Input: part model. Units: mm. Frame: model coordinates. Face numbers are marked on the shaded views. A direction names the side the tool comes from. Give positions to 0.01 mm unless a question says otherwise; leave off trailing zeros. Write each loop counter-clockwise with the first axis right and the second up, starting at its lowest first coordinate (ties: lowest second). Pieces come first, ordered by that corner, then holes. Notation, with made-up numbers: (43, 60.5) - (56, 60.5) arc R24 cw to (56, 70.5) - close; hole circle Ø7 at (-36, 83.5). An arc over 180 degrees is marked (long way). Use a Markdown table: item, result. Add a question column.
1. Set-up query: the marked faces 1 and 2. Return all of +Z, -Z, +X, -X, +Y, -Y with unobstructed straight access to the full face (end or side cutting, diameter ignored); none if empty.
2. Pin query (flat end, axial travel): pin 1 (10.5 mm diameter, centred on x = -90.93, y = 52.5, fed in from +Z); pin 2 (5 mm diameter, centred on x = 50.5, z = 10.5, fed in from -Y); pin 3 (17 mm diameter, centred on x = 0, y = 105, fed in from +Z); pin 4 (4 mm diameter, centred on y = -31.5, z = 7.5, fed in from +X). Return the tip coordinate at first contact, or that it passes through.
3. Section query B-B, the plane x = -91. Return loops of the section in (y, z).
4. Section query D-D, the plane z = 1. Return loops of the section in (x, y), plus the area to 3 significant figures.
5. Mould query, pull axis X, two halves, no side actions, for the marked faces 3, 4 and 5. Classes: released by +X, released by -X, zero draft, split by the parting line, or undercut.
6. Section query C-C, the plane y = -105. Return loops of the section in (x, z), plus the area to 3 significant figures.
7. Material intervals for probe 1 along Y at (x, z) = (0, -1.75); probe 2 along Z at (x, y) = (-73.5, 66.5); probe 3 along Z at (x, y) = (-5, 78.5), sorted ascending.
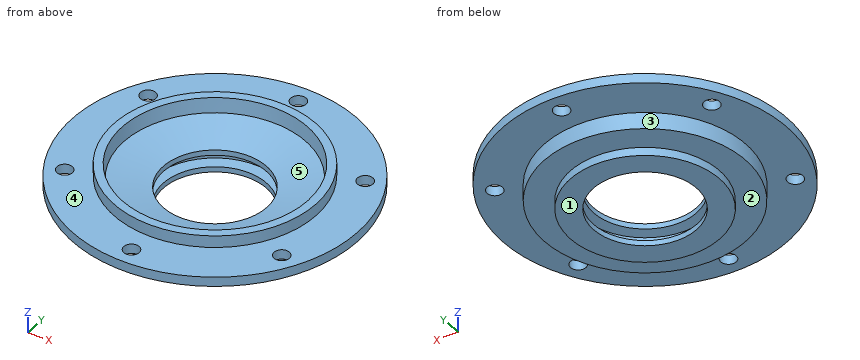
```python
from build123d import *

# Parameters (mm, degrees)
SKETCH_2_R               = 6.5
CUT_EXTRUDE_1_DEPTH      = 172
PATTERN_CIRCULAR_1_COUNT = 6


with BuildPart() as part:
    # 草图1 → 旋转1 (revolve)
    with BuildSketch(Plane(origin=(0, 0, 0), x_dir=(0, 0, -1), z_dir=(1, 0, 0)), mode=Mode.PRIVATE) as revolve_1_sk:
        Polygon((-9.5, 43.5), (-5, 43.5), (-4, 52.5), (4, 52.5), (5, 43.5), (9.5, 43.5), (9.5, 63), (2.5, 63), (2.5, 85), (-11.5, 85), (-11.5, 120), (-19.5, 120), (-19.5, 85), (-29.5, 85), (-29.5, 78), (-17.5, 76.5), align=None)
    revolve(revolve_1_sk.sketch.rotate(Axis((0, 0, 1000), (0, 0, -1)), 90), axis=Axis((0, 0, 1000), (0, 0, -1)))

    # 草图2 → 切除-拉伸1 (cut, through all)
    with BuildSketch(Plane(origin=(0, 0, 11.5), x_dir=(-1, 0, 0), z_dir=(0, 0, -1))):
        with Locations((0, 105)):
            Circle(SKETCH_2_R)
    cut_extrude_1 = extrude(amount=-CUT_EXTRUDE_1_DEPTH, mode=Mode.SUBTRACT)

    # 阵列(圆周)1: 切除-拉伸1 ×6 about axis
    pattern_circular_1_axis = Axis((0, 0, 0), (0, 0, 1))
    for i in range(1, PATTERN_CIRCULAR_1_COUNT):
        add(cut_extrude_1.rotate(pattern_circular_1_axis, i * 360 / PATTERN_CIRCULAR_1_COUNT), mode=Mode.SUBTRACT)


solid = part.part
```
Result sheet:
| question | item | result |
|---|---|---|
| 1 | face 1 | -Z, +X, -X, +Y, -Y |
| 1 | face 2 | -Z |
| 2 | pin 1 | passes through |
| 2 | pin 2 | stops at y = -109.89 |
| 2 | pin 3 | stops at z = 19.5 |
| 2 | pin 4 | stops at x = 79.72 |
| 3 | outline | (-78.22, 11.5) - (-59, 11.5) - (-59, 19.5) - (-78.22, 19.5) - close; (-46, 11.5) - (46, 11.5) - (46, 19.5) - (-46, 19.5) - close; (59, 11.5) - (78.22, 11.5) - (78.22, 19.5) - (59, 19.5) - close |
| 4 | outline | circle Ø170 at (0, 0); hole circle Ø105 at (0, 0) |
| 4 | area | 14,000 mm² |
| 5 | face 3 | split by the parting line |
| 5 | face 4 | zero draft |
| 5 | face 5 | undercut |
| 6 | outline | (-58.09, 11.5) - (-6.5, 11.5) - (-6.5, 19.5) - (-58.09, 19.5) - close; (6.5, 11.5) - (58.09, 11.5) - (58.09, 19.5) - (6.5, 19.5) - close |
| 6 | area | 826 mm² |
| 7 | probe 1 | y = -85 to -52.5, 52.5 to 85 |
| 7 | probe 2 | z = 11.5 to 19.5 |
| 7 | probe 3 | z = -2.5 to 29.5 |
